Build history of the part. All positions in model axes, mm. A direction names the side the tool comes from. Coordinates: 2 decimals unless noted, no trailing zeros. Order: outer loops, then holes, each group sorted by start corner. A loop starts at its lowest first (then second) coordinate and runs counter-clockwise, first axis right, second up. Notation, with made-up numbers: (63.5, -0.75) - (116.5, -0.75) arc R21 cw to (116.5, 17.25) - close; hole circle Ø1 at (-38.75, 16.5). An arc over 180 degrees is marked (long way). Answer as CSV lines item,"result". Start each with the question number.
from build123d import *

# Parameters (mm, degrees)
SKETCH_2_R          = 1.6
CUT_EXTRUDE_1_DEPTH = 22.136461388
CUT_EXTRUDE_START   = -4
SKETCH_2_4_R        = 1.6
CUT_EXTRUDE_2_DEPTH = 2.7


with BuildPart() as part:
    # Sketch 1 → Revolve 1 (revolve)
    with BuildSketch(Plane(origin=(0, 0, 0), x_dir=(0, 0, -1), z_dir=(1, 0, 0)), mode=Mode.PRIVATE) as revolve_1_sk:
        Polygon((0, 11.5), (0, 1.5), (8, 1.5), (8, 7), (13.5, 7), (13.5, 11.5), (12, 11.5), (12, 10), (1.5, 10), (1.5, 11.5), align=None)
    revolve(revolve_1_sk.sketch.rotate(Axis((0, 0, 0), (0, 0, -1)), 90), axis=Axis((0, 0, 0), (0, 0, -1)))

    # Sketch 2 → Cut-Extrude 1 (cut, through all)
    with BuildSketch(Plane(origin=(0, 0, 0), x_dir=(1, 0, 0), z_dir=(0, 1, 0))):
        with Locations(Location((0, 4, 0), (0, 0, 270))):
            Circle(SKETCH_2_R)
    cut_extrude_1 = extrude(amount=-CUT_EXTRUDE_1_DEPTH, mode=Mode.SUBTRACT)

    # Sketch 2_4 → Cut-Extrude 2 (cut)
    with BuildSketch(Plane(origin=(0, 0, 0), x_dir=(1, 0, 0), z_dir=(0, 1, 0)).offset(CUT_EXTRUDE_START)):
        Polygon((-2.85, 0), (2.85, 0), (2.85, 2.354551733), (2.85, 5.645448267), (0, 7.290896534), (-2.85, 5.645448267), (-2.85, 2.354551733), align=None)
        with Locations(Location((0, 4, 0), (0, 0, 270))):
            Circle(SKETCH_2_4_R, mode=Mode.SUBTRACT)
    cut_extrude_2 = extrude(amount=-CUT_EXTRUDE_2_DEPTH, mode=Mode.SUBTRACT)

    # Mirror 1: Cut-Extrude 1, Cut-Extrude 2 across plane
    add(cut_extrude_1.mirror(Plane.ZX), mode=Mode.SUBTRACT)
    add(cut_extrude_2.mirror(Plane.ZX), mode=Mode.SUBTRACT)


solid = part.part
(1) Band-saw the part on C-C on z = -4. List the corners of the cut face in (x, y), plus the area to 3 significant figures.
(2) Band-saw the part on A-A on y = 0. List the corners of the cut face in (x, z).
(3) Band-saw the part on D-D on x = 5.5. List the corners of the cut face in (y, z), plus the area to 3 significant figures.
(4) Probe L1, parallel to Y at x = 0, z = -0.5; L2, parallel to Z at x = 0, y = 9.1; L3, parallel to Y at x = -2.75, z = -5.25. List the from-to ranges inside material, lowest first. Write a range as [from, to].
(5) Pull direction Y, two halves, no side cores. Call faces 1 (the flat face through (0, -2, -8)), 2 (the cylindrical face through (-1.5, -11.4, -12.7)), 3 (the flat face through (-9, -5, -12)): +Y half, -Y half, draft (parallel to the pull), parting line (faces both ways), or undercut.
(6) Which spindle directions (+Z, -Z, +X, -X, +Y, -Y) get a long thin tool onto all of the face, cutting with end or side? Do faces 4 (the cylindrical face through (1.386, 0.575, -1.363)), 5 (the flat face through (9, -5, -1.5)), 6 (the flat face through (2, 0, 0)), 7 (the cylindrical face through (3.23, 6.21, -10.79)), 8 (the flat face through (0, 4, -2)). Say none if no direction does.
(7) Band-saw the part on B-B on y = 2.5. List the corners of the cut face in (x, z), plus the area to 3 significant figures.
(8) Drop flat-ended pins along their axis: pin 1 Ø6 at (x, y) = (-1, -1) entering from -Z; pin 2 Ø3 at (y, z) = (-5, -2) entering from +X; pin 3 Ø0.8 at (y, z) = (-5, -3.5) entering from -X; pin 4 Ø12 at (x, y) = (-9, -8.5) entering from -Z. Give the stop position or say it passes through.
Filled in:
1,outline,"(-2.85, -6.7) - (-2.85, -4) - (-1.6, -4) - (-1.6, 4) - (-2.85, 4) - (-2.85, 6.7) - (-1.6, 6.7) - (-1.6, 9.87) arc R10 ccw to (-1.6, -9.87) - (-1.6, -6.7) - close; (1.6, -9.87) arc R10 ccw to (1.6, 9.87) - (1.6, 6.7) - (2.85, 6.7) - (2.85, 4) - (1.6, 4) - (1.6, -4) - (2.85, -4) - (2.85, -6.7) - (1.6, -6.7) - close"
1,area,"237 mm^2"
2,outline,"(-11.5, -13.5) - (-7, -13.5) - (-7, -8) - (-1.5, -8) - (-1.5, -4.56) arc R1.6 cw to (-1.5, -3.44) - (-1.5, 0) - (-11.5, 0) - (-11.5, -1.5) - (-10, -1.5) - (-10, -12) - (-11.5, -12) - close; (1.5, -8) - (7, -8) - (7, -13.5) - (11.5, -13.5) - (11.5, -12) - (10, -12) - (10, -1.5) - (11.5, -1.5) - (11.5, 0) - (1.5, 0) - (1.5, -3.44) arc R1.6 cw to (1.5, -4.56) - close"
3,outline,"(-10.1, -13.5) - (-4.33, -13.5) - (-4.33, -8) - (4.33, -8) - (4.33, -13.5) - (10.1, -13.5) - (10.1, -12) - (8.35, -12) - (8.35, -1.5) - (10.1, -1.5) - (10.1, 0) - (-10.1, 0) - (-10.1, -1.5) - (-8.35, -1.5) - (-8.35, -12) - (-10.1, -12) - close"
3,area,"188 mm^2"
4,L1,"y = [-11.5, -6.7], [-4, -1.5], [1.5, 4], [6.7, 11.5]"
4,L2,"z = [-13.5, -5.6], [-2.4, 0]"
4,L3,"y = [-9.61, -6.7], [-4, 4], [6.7, 9.61]"
5,face 1,"undercut"
5,face 2,"parting line"
5,face 3,"draft"
6,face 4,"+Z, -Z"
6,face 5,"none"
6,face 6,"+Z, +X, -X, +Y, -Y"
6,face 7,"-Z"
6,face 8,"+Z"
7,outline,"(-11.22, -13.5) - (-6.54, -13.5) - (-6.54, -8) - (6.54, -8) - (6.54, -13.5) - (11.22, -13.5) - (11.22, -12) - (9.68, -12) - (9.68, -1.5) - (11.22, -1.5) - (11.22, 0) - (-11.22, 0) - (-11.22, -1.5) - (-9.68, -1.5) - (-9.68, -12) - (-11.22, -12) - close; hole circle Ø3.2 at (0, -4)"
7,area,"191 mm^2"
8,pin 1,"stops at z = -8"
8,pin 2,"stops at x = 10.93"
8,pin 3,"stops at x = -8.88"
8,pin 4,"stops at z = -13.5"
